Input: part model. Units: mm. Frame: model coordinates. A direction names the side the tool comes from. Coordinates: 2 decimals unless noted, no trailing zeros. Order: outer loops, then holes, each group sorted by start corner. A loop starts at its lowest first (then second) coordinate and runs counter-clockwise, first axis right, second up. Notation, with made-up numbers: M -27,-34 L 11,-34 A5 ccw 11,-29 Z; hole C 36,49.25 d4. An arc over 180 degrees is marked long. Answer in a Markdown table with one row per item.
from build123d import *

# Parameters (mm, degrees)
SKETCH2_R           = 2.3
SKETCH2_R_2         = 1.7
BOSS_EXTRUDE1_DEPTH = 5
BOSS_EXTRUDE2_DEPTH = 5
SKETCH4_W           = 60.3
SKETCH4_H           = 15
BOSS_EXTRUDE3_DEPTH = 50
SKETCH5_R           = 1.7
SKETCH5_R_2         = 7.5
BOSS_EXTRUDE4_DEPTH = 5
SKETCH7_W           = 60.3
SKETCH7_H           = 50
BOSS_EXTRUDE6_DEPTH = 7


with BuildPart() as part:
    # Sketch2 → Boss-Extrude1 (new body)
    with BuildSketch(Plane(origin=(0, 0, 0), x_dir=(1, 0, 0), z_dir=(0, 1, 0))):
        with BuildLine():
            Line((15.15, -32.7), (-15.15, -32.7))
            ThreePointArc((-15.15, -32.7), (-25.756601718, -28.306601718), (-30.15, -17.7))
            Line((-30.15, -17.7), (-30.15, 17.7))
            ThreePointArc((-30.15, 17.7), (-25.756601718, 28.306601718), (-15.15, 32.7))
            Line((-15.15, 32.7), (15.15, 32.7))
            ThreePointArc((15.15, 32.7), (25.756601718, 28.306601718), (30.15, 17.7))
            Line((30.15, 17.7), (30.15, -17.7))
            ThreePointArc((30.15, -17.7), (25.756601718, -28.306601718), (15.15, -32.7))
        make_face()
        with Locations(Location((-15, 20, 0), (0, 0, 270))):
            Circle(SKETCH2_R, mode=Mode.SUBTRACT)
        with Locations(Location((-25, 0, 0), (0, 0, 270))):
            Circle(SKETCH2_R, mode=Mode.SUBTRACT)
        with Locations(Location((-15, -20, 0), (0, 0, 270))):
            Circle(SKETCH2_R, mode=Mode.SUBTRACT)
        with Locations(Location((-22.5, -15, 0), (0, 0, 270))):
            Circle(SKETCH2_R_2, mode=Mode.SUBTRACT)
        with Locations(Location((-22.5, 15, 0), (0, 0, 270))):
            Circle(SKETCH2_R_2, mode=Mode.SUBTRACT)
        with Locations(Location((15, 20, 0), (0, 0, 90))):
            Circle(SKETCH2_R, mode=Mode.SUBTRACT)
        with Locations(Location((22.5, 15, 0), (0, 0, 90))):
            Circle(SKETCH2_R_2, mode=Mode.SUBTRACT)
        with Locations(Location((25, 0, 0), (0, 0, 90))):
            Circle(SKETCH2_R, mode=Mode.SUBTRACT)
        with Locations(Location((22.5, -15, 0), (0, 0, 90))):
            Circle(SKETCH2_R_2, mode=Mode.SUBTRACT)
        with Locations(Location((15, -20, 0), (0, 0, 90))):
            Circle(SKETCH2_R, mode=Mode.SUBTRACT)
        with BuildLine():
            Line((-9, 4.716333345), (-9, -16.9))
            Line((-9, -16.9), (9, -16.9))
            Line((9, -16.9), (9, 4.716333345))
            ThreePointArc((9, 4.716333345), (0, 19.4), (-9, 4.716333345))
        make_face(mode=Mode.SUBTRACT)
    extrude(amount=BOSS_EXTRUDE1_DEPTH)

    # Sketch3 → Boss-Extrude2 (add)
    with BuildSketch(Plane.XZ):
        Polygon((-30.15, 17.7), (-30.15, 42.3), (30.15, 42.3), (30.15, 17.7), (15.15, 32.7), (-15.15, 32.7), align=None)
    extrude(amount=-BOSS_EXTRUDE2_DEPTH)

    # Sketch4 → Boss-Extrude3 (add)
    with BuildSketch(Plane(origin=(0, 5, 0), x_dir=(1, 0, 0), z_dir=(0, 1, 0))):
        with Locations((0, -34.8)):
            Rectangle(SKETCH4_W, SKETCH4_H)
    extrude(amount=BOSS_EXTRUDE3_DEPTH)

    # Sketch5 → Boss-Extrude4 (add)
    with BuildSketch(Plane(origin=(0, 55, 0), x_dir=(1, 0, 0), z_dir=(0, 1, 0))):
        with BuildLine():
            Line((-30.15, -42.3), (30.15, -42.3))
            Line((30.15, -42.3), (30.15, 17.7))
            ThreePointArc((30.15, 17.7), (25.756601718, 28.306601718), (15.15, 32.7))
            Line((15.15, 32.7), (-15.15, 32.7))
            ThreePointArc((-15.15, 32.7), (-25.756601718, 28.306601718), (-30.15, 17.7))
            Line((-30.15, 17.7), (-30.15, -42.3))
        make_face()
        with Locations(Location((-22.5, 15, 0), (0, 0, 270))):
            Circle(SKETCH5_R, mode=Mode.SUBTRACT)
        with Locations(Location((-22.5, -15, 0), (0, 0, 270))):
            Circle(SKETCH5_R, mode=Mode.SUBTRACT)
        with Locations(Location((22.5, 15, 0), (0, 0, 90))):
            Circle(SKETCH5_R, mode=Mode.SUBTRACT)
        with Locations(Location((22.5, -15, 0), (0, 0, 90))):
            Circle(SKETCH5_R, mode=Mode.SUBTRACT)
        with Locations(Location((0, 9.3, 0), (0, 0, 270))):
            Circle(SKETCH5_R_2, mode=Mode.SUBTRACT)
    extrude(amount=BOSS_EXTRUDE4_DEPTH)

    # Sketch7 → Boss-Extrude6 (add)
    with BuildSketch(Plane(origin=(0, 0, 27.3), x_dir=(-1, 0, 0), z_dir=(0, 0, -1))):
        with Locations((0, 30)):
            Rectangle(SKETCH7_W, SKETCH7_H)
    extrude(amount=BOSS_EXTRUDE6_DEPTH)


solid = part.part
1) Cut plane B-B, the plane z = -9.3. Output: boundary loops of the cut face in (x, y).
Resolved:
| item | result |
|---|---|
| outline | M -30.15,0 L -10.1,0 L -10.1,5 L -30.15,5 Z; M -30.15,55 L -7.5,55 L -7.5,60 L -30.15,60 Z; M 7.5,55 L 30.15,55 L 30.15,60 L 7.5,60 Z; M 10.1,0 L 30.15,0 L 30.15,5 L 10.1,5 Z |
2) Mould query, pull axis Y, two halves, no side actions, for faces 3 (the face through (0, 55, -1)), 4 (the face through (-15, 5, 21)), 5 (the face through (7, 5, -18)), 6 (the face through (-14.309, 2.465, -17.806)). Classes: +Y half, -Y half, draft (parallel to the pull), parting line (faces both ways), or undercut.
Resolved:
| item | result |
|---|---|
| face 3 | undercut |
| face 4 | -Y half |
| face 5 | undercut |
| face 6 | draft |
3) Cut plane A-A, the plane z = 4.5. Output: boundary loops of the cut face in (x, y).
Resolved:
| item | result |
|---|---|
| outline | M -30.15,0 L -9,0 L -9,5 L -30.15,5 Z; M -30.15,55 L 30.15,55 L 30.15,60 L -30.15,60 Z; M 9,0 L 30.15,0 L 30.15,5 L 9,5 Z |
4) Cut plane D-D, the plane y = 37. Output: boundary loops of the cut face in (x, z).
Resolved:
| item | result |
|---|---|
| outline | M -30.15,20.3 L 30.15,20.3 L 30.15,42.3 L -30.15,42.3 Z |
5) Reachability of faces 1 (the face through (30.15, 30, 26)), 2 (the face through (9, 2, 6)) from +Z, -Z, +X, -X, +Y, -Y: full face, straight path, thin tool, end or side. Return the list, or none.
Resolved:
| item | result |
|---|---|
| face 1 | +Z, -Z, +X, +Y, -Y |
| face 2 | -Y |
6) Contact query for flat-ended pins moving along their axis: pin 1 (1 mm diameter, centred on x = 3.5, z = 10, fed in from -Y); pin 2 (3 mm diameter, centred on x = -0.5, y = 15, fed in from -Z); pin 3 (5 mm diameter, centred on y = 19.5, z = 18.5, fed in from -X). Output: stop coordinate, or through.
Resolved:
| item | result |
|---|---|
| pin 1 | stops at y = 55 |
| pin 2 | stops at z = 20.3 |
| pin 3 | stops at x = -30.15 |
7) Cut plane C-C, the plane x = 4. Output: boundary loops of the cut face in (y, z).
Resolved:
| item | result |
|---|---|
| outline | M 0,-32.7 L 5,-32.7 L 5,-18.57 L 0,-18.57 Z; M 0,16.9 L 5,16.9 L 5,20.3 L 55,20.3 L 55,-2.96 L 60,-2.96 L 60,42.3 L 0,42.3 Z; M 55,-32.7 L 60,-32.7 L 60,-15.64 L 55,-15.64 Z |
8) Material intervals for probe 1 along X at (y, z) = (2.35, 15); probe 2 along X at (y, z) = (3, 0); probe 3 along Y at (x, z) = (21.5, 1), sorted ascending.
Resolved:
| item | result |
|---|---|
| probe 1 | x = -30.15 to -24.2, -20.8 to -9, 9 to 20.8, 24.2 to 30.15 |
| probe 2 | x = -30.15 to -27.3, -22.7 to -9, 9 to 22.7, 27.3 to 30.15 |
| probe 3 | y = 0 to 5, 55 to 60 |
